Geometry: see drawing. Coordinates: mm, zero at the bounding-box minimum. A direction names the side the tool comes from. Give positions to 0.01 mm unless a question says otherwise; leave off trailing zeros. Write each loop counter-clockwise with the first axis right and the second up, starting at its lowest first coordinate (ties: lowest second). Pieces come first, ordered by that corner, then holes. Notation, with made-up numbers: (60, 46.25) -> (101, 46.25) arc R8 ccw to (101, 56.25) -> close; hole circle Ø7 at (45, -16.75). An arc over 180 degrees is marked (long way). Use one line per item in the form item = value. Start each with the question number.
(1) Cut plane A-A, the plane y = 60. Output: boundary loops of the cut face in (x, z).
(2) Material intervals for line 1 along Z through (x, y) = (106.5, 27); line 2 along Z through (x, y) = (83.5, 53); line 3 along X through (y, z) = (13, 88), sorted ascending. Write a range as from..to.
(3) Cut plane D-D, the plane z = 23.5. Output: boundary loops of the cut face in (x, y).
(4) Set-up query: the marked faces 1 and 2. Return all of +Z, -Z, +X, -X, +Y, -Y with unobstructed straight access to the full face (end or side cutting, diameter ignored); none if empty.
(5) Cut plane C-C, the plane z = 121. Output: boundary loops of the cut face in (x, y).
(6) First-contact query: P1, Ø1, axis at x = 72, y = 12, coming from the -Z side; P2, Ø8, axis at x = 55, z = 142.5, coming from the +Y side; P3, Ø1, axis at y = 19.5, z = 203, coming from the +X side; P4, Ø5, axis at y = 61.5, z = 93.5, coming from the -X side. Flat tips, straight axial feed; report the tip coordinate or a pass-through.
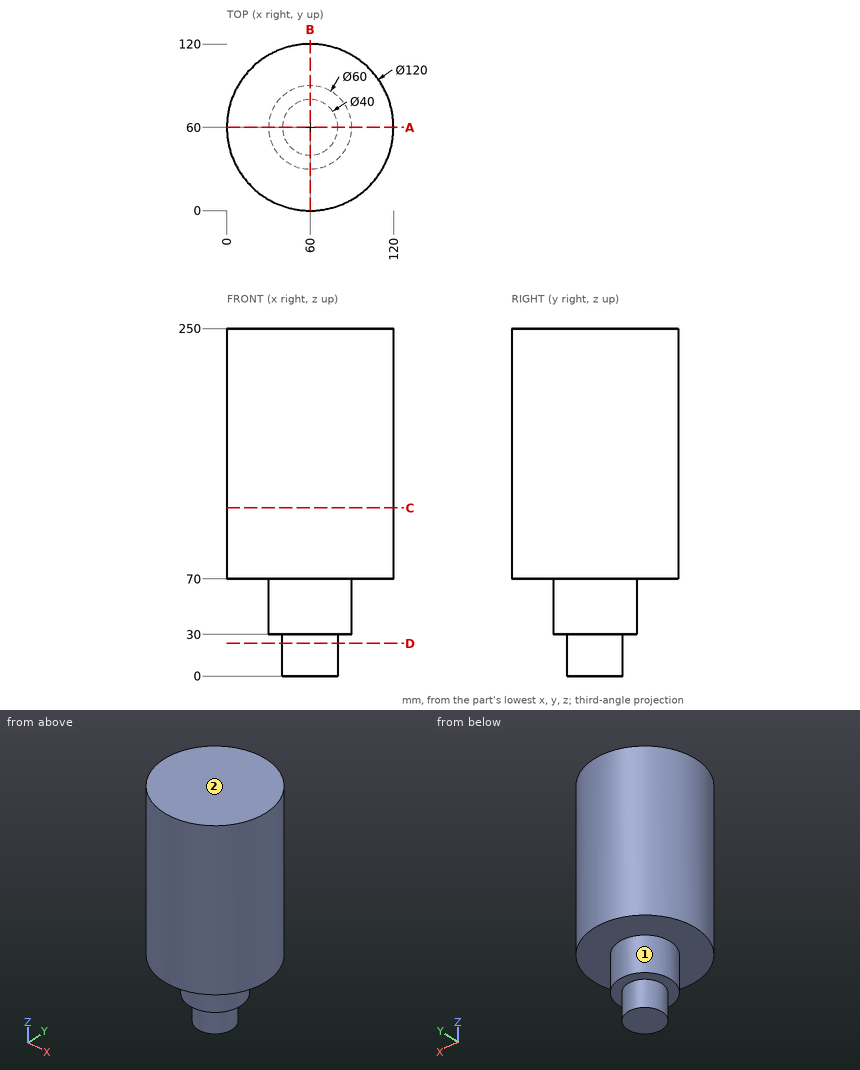
Geometry says:
q1.outline = (0, 70) -> (30, 70) -> (30, 30) -> (40, 30) -> (40, 0) -> (80, 0) -> (80, 30) -> (90, 30) -> (90, 70) -> (120, 70) -> (120, 250) -> (0, 250) -> close
q2.line_1 = 70..250
q2.line_2 = 30..250
q2.line_3 = 22.7..97.3
q3.outline = circle Ø40 at (60, 60)
q4.face_1 = -Z
q4.face_2 = +Z, +X, -X, +Y, -Y
q5.outline = circle Ø120 at (60, 60)
q6.P1 = 70
q6.P2 = 119.99
q6.P3 = 104.72
q6.P4 = 0
